Autodesk Inventor part; units mm, degrees
ref_plane "Work Plane2" through (0, 11, 0) normal (0, 1, 0) x (-1, 0, 0)
ref_plane "Work Plane4" through (9.75, 13.75, 26.5) normal (0, 0, 1) x (1, 0, 0)
ref_plane "YZ Plane" through (0, 0, 0) normal (1, 0, 0) x (0, 1, 0)
sketch "Sketch1" plane through (0, 0, 0) normal (0, 0, 1) x (1, 0, 0)
  line L0 (0, 0) -> (25, 0)
  line L1 (25, 0) -> (25, 22)
  line L2 (25, 22) -> (0, 22)
  line L3 (0, 22) -> (0, 0)
  dimension "d0" = 25
  dimension "d1" = 22
extrude "Extrusion1" add sketch "Sketch1" along normal blind 5
sketch "Sketch2" plane through (0, 0, 5) normal (0, 0, 1) x (1, 0, 0)
  circle A0 centre (9, 8.25) radius 1.45
  line L0 (0, 0) -> (25, 0)
  line L1 (0, 22) -> (0, 0)
  dimension "d6" = 2.9
  dimension "d7" = 8.25
  dimension "d8" = 9
extrude "Extrusion2" add sketch "Sketch2" along normal blind 2
sketch "Sketch3" plane through (0, 0, 5) normal (0, 0, 1) x (1, 0, 0)
  line L0 (17.5, 5.5) -> (19.5, 5.5)
  line L1 (19.5, 5.5) -> (19.5, 16.5)
  line L2 (19.5, 16.5) -> (17.5, 16.5)
  line L3 (17.5, 16.5) -> (17.5, 5.5)
  line L4 (0, 0) -> (25, 0)
  line L5 (0, 22) -> (0, 0)
  circle A0 centre (9, 8.25) radius 1.45 construction
  dimension "d9" = 2
  dimension "d10" = 11
  dimension "d58" = 8.5
  dimension "d59" = 2.75
extrude "Extrusion3" cut sketch "Sketch3" against normal blind 1
sketch "Sketch4" plane through (0, 0, 5) normal (0, 0, 1) x (1, 0, 0)
  line L0 (0, 22) -> (25, 22)
  line L1 (25, 22) -> (25, 17)
  line L2 (25, 17) -> (0, 17)
  line L3 (0, 17) -> (0, 22)
  line L4 (25, 0) -> (25, 22) construction
  line L5 (25, 17) -> (20, 17)
  line L6 (20, 17) -> (20, 0)
  line L7 (20, 0) -> (25, 0)
  line L8 (25, 0) -> (25, 17)
  line L9 (0, 0) -> (25, 0)
  line L10 (20, 0) -> (0, 0)
  line L11 (0, 0) -> (0, 5)
  line L12 (0, 5) -> (20, 5)
  line L13 (20, 5) -> (20, 0)
  line L14 (0, 22) -> (0, 0)
  line L15 (0, 5) -> (5, 5)
  line L16 (5, 5) -> (5, 17)
  line L17 (5, 17) -> (0, 17)
  line L18 (0, 17) -> (0, 5)
  dimension "d16" = 5
  dimension "d17" = 5
  dimension "d18" = 5
  dimension "d19" = 5
extrude "Extrusion4" add sketch "Sketch4" along normal blind 4 contours L0 L1 L2 L3 | L2 L16 L12 L14 | L8 L7 L6 L2 | L12 L6 L9 L11
ref_plane "Work Plane2" through (0, 11, 0) normal (0, 1, 0) x (-1, 0, 0)
sketch "Sketch15" plane through (0, 0, 9) normal (0, 0, 1) x (1, 0, 0)
  line L0 (25, 22) -> (0, 22)
  line L1 (0, 22) -> (0, 0)
  line L2 (0, 0) -> (25, 0)
  line L3 (25, 0) -> (25, 22)
extrude "Extrusion15" add sketch "Sketch15" along normal blind 5
sketch "Sketch18" plane through (0, 0, 14) normal (0, 0, 1) x (1, 0, 0)
  circle A0 centre (9.75, 13.75) radius 2
  circle A1 centre (9, 8.25) radius 1.45 construction
  point P0 (0, 0)
  dimension "d70" = 4
  dimension "d107" = 5.5
  dimension "d108" = 0.75
extrude "Extrusion17" add sketch "Sketch18" along normal blind 10
fillet "Fillet5" radius 4 1 edges at (7.75, 13.75, 14)
fillet "Fillet6" radius 4 8 edges at (0, 11, 14) (12.5, 0, 14) (25, 11, 14) (12.5, 22, 14) (0, 0, 7) (25, 0, 7) (0, 22, 7) (25, 22, 7)
ref_plane "Work Plane4" through (9.75, 13.75, 26.5) normal (0, 0, 1) x (1, 0, 0)
sketch "Sketch21" plane through (9.75, 13.75, 26.5) normal (0, 0, 1) x (1, 0, 0)
  circle A0 centre (0, 0) radius 2 construction
  circle A1 centre (0, 0) radius 2.25
  point P0 (-9.75, -13.75)
  dimension "d91" = 0.25
loft "Loft3" add profiles "Sketch21" section 2 edges at (7.75, 13.75, 24)
fillet "Fillet8" radius 0.25 1 edges at (7.5, 13.75, 26.5)
fillet "Fillet9" radius 2 1 edges at (7.75, 13.75, 24)
sketch "Sketch22" plane through (9.75, 13.75, 26.5) normal (0, 0, 1) x (1, 0, 0)
  circle A0 centre (0, 0) radius 0.75
  point P0 (-9.75, -13.75)
  dimension "d98" = 1.5
extrude "Extrusion19" cut sketch "Sketch22" against normal blind 20
sketch "Sketch23" plane through (25, 4, 0) normal (1, 0, 0) x (0, 0, -1)
  line L0 (-9, 13) -> (-9, 1) construction
  line L1 (-5.75, 4.75) -> (-5.75, 9.25)
  line L2 (-7.5, 4.75) -> (-7.5, 9.25)
  line L3 (-5.75, 4.75) -> (-7.5, 4.75)
  line L4 (-5, 1.5) -> (-5, 12.5)
  line L5 (-7.5, 9.25) -> (-5.75, 9.25)
  point P0 (0, -4)
  point P1 (-9, 7)
  point P2 (-9, 7)
  dimension "d104" = 4.5
  dimension "d111" = 1.5
  dimension "d112" = 1.75
extrude "Extrusion20" cut sketch "Sketch23" against normal blind 5
fillet "Fillet10" radius 3.5 2 edges at (12.5, 17, 9) (12.5, 5, 9)
fillet "Fillet11" radius 3 5 edges at (5, 15.9749, 7.9749) (5, 17, 5.25) (5, 6.0251, 7.9749) (5, 5, 5.25) (5, 11, 9)
equation "\"d17\" = d16"
equation "\"d18\" = d16"
equation "\"d19\" = d16"
properties part number "DAQcapsule"
Design review of the part built by this model. Coordinates are the model's own, in mm. A direction names the side the tool comes from. Coordinates: 2 decimals unless noted, no trailing zeros. Order: outer loops, then holes, each group sorted by start corner. A loop starts at its lowest first (then second) coordinate and runs counter-clockwise, first axis right, second up.
1) Wall thickness on line 1 along Y through (x, z) = (9.75, 21.5); line 2 along Z through (x, y) = (15.75, 9); line 3 along Z through (x, y) = (7, 10): over which ranges is each line inside the solid? List them lowest first.
2) Mouldability with a two-part tool opening along Y and no side actions: class faces 1 (the flat face through (23, 13.25, 7)), 2 (the flat face through (13, 22, 5)), 3 (the conical face through (8.088, 12.476, 24.941)) as +Y half, -Y half, draft (parallel to the pull), parting line (faces both ways), or undercut.
3) Take a section at B-B, the plane y = 1.75. Give the boundary of the cut face in (x, z).
4) For faces 4 (the flat face through (4.4, 17.3, 14)), 5 (the cylindrical face through (14.08, 16, 7.95)), 6 (the flat face through (23, 8.75, 7)), 7 (the cylindrical face through (1.203, 16.714, 12.859)), 8 (the flat face through (12, 11, 0)), list the 3-axis set-ups (+Z, -Z, +X, -X, +Y, -Y) from which the entire face can be reached by the end or side of a thin tool; tool diameter is ignored.
5) Clearance check with flat-ended pins moving along their axes: pin 1 (4.5 mm diameter, centred on y = 12.5, z = 7.5, fed in from -X); pin 2 (1.9 mm diameter, centred on x = 22.5, z = 6.5, fed in from -Y); pin 3 (5 mm diameter, centred on x = 21.5, y = 10.5, fed in from +Z); pin 4 (1.4 mm diameter, centred on x = 9.75, y = 13.75, fed in from +Z). State where each tip first meets the part, or that it passes through.
6) Take a section at A-A, the plane x = 19. Give the boundary of the cut face in (y, z), and give its area (3 significant figures).
Returned:
1. line 1: y = 11.75 to 13, 14.5 to 15.75
1. line 2: z = 0 to 5, 9 to 14
1. line 3: z = 0 to 5, 8.83 to 14.23
2. face 1: undercut
2. face 2: +Y half
2. face 3: parting line
3. outline: (0.69, 0) - (24.31, 0) - (24.31, 10) arc R3.31 ccw to (21, 13.31) - (4, 13.31) arc R3.31 ccw to (0.69, 10) - close
4. face 4: +Z, -X, +Y
4. face 5: none
4. face 6: +X
4. face 7: +Z, -X, +Y, -Y
4. face 8: -Z, +X, -X, +Y, -Y
5. pin 1: stops at x = 0
5. pin 2: stops at y = 0.04
5. pin 3: stops at z = 14
5. pin 4: stops at z = 5
6. outline: (0, 0) - (22, 0) - (22, 10) arc R4 ccw to (18, 14) - (4, 14) arc R4 ccw to (0, 10) - close; hole (5, 5) - (5.5, 5) - (5.5, 4) - (16.5, 4) - (16.5, 5) - (17, 5) - (17, 5.5) arc R3.5 ccw to (13.5, 9) - (8.5, 9) arc R3.5 ccw to (5, 5.5) - close
6. area: 247 mm2
